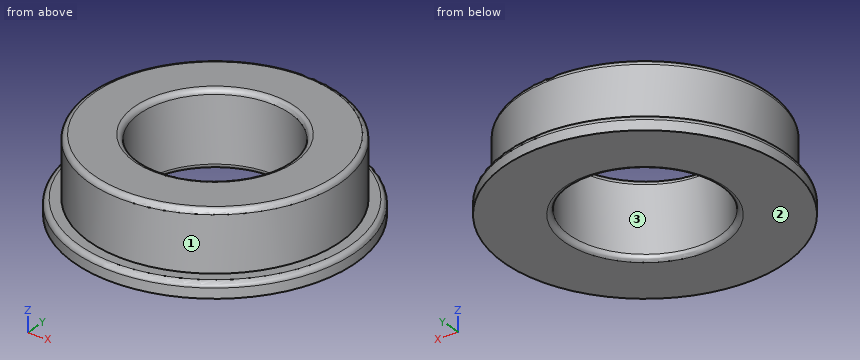
Autodesk Inventor part; units mm, degrees
ref_plane "YZ Plane" through (0, 0, 0) normal (1, 0, 0) x (0, 1, 0)
ref_plane "XZ Plane" through (0, 0, 0) normal (0, 1, 0) x (-1, 0, 0)
ref_plane "XY Plane" through (0, 0, 0) normal (0, 0, 1) x (1, 0, 0)
sketch "Sketch1" plane through (0, 0, 0) normal (0, 0, 1) x (1, 0, 0)
  circle A0 centre (0, 0) radius 3
  circle A1 centre (0, 0) radius 5
  circle A2 centre (0, 0) radius 5.6
  dimension "d0" = 6
  dimension "d1" = 10
  dimension "d2" = 11.2
extrude "Extrusion1" add sketch "Sketch1" along normal blind 3 contours A1
extrude "Extrusion2" add sketch "Sketch1" along normal blind 0.6 contours A2
fillet "Fillet1" radius 0.2 4 edges at (-5.6, 0, 0.6) (-5, 0, 3) (-3, 0, 3) (-3, 0, 0)
properties part number "flange_bearing"
Verification items for the finished model (mm, model axes). Face numbers are marked on the shaded views. Give positions to 0.01 mm unless a question says otherwise; leave off trailing zeros. Order: outer loops, then holes, each group sorted by start corner. A loop starts at its lowest first (then second) coordinate and runs counter-clockwise, first axis right, second up. Notation, with made-up numbers: (52, 39.5) -> (107, 39.5) arc R27 cw to (107, 59.5) -> close; hole circle Ø10 at (-6.5, -19). An arc over 180 degrees is marked (long way). Use a Markdown table: item, result.
1) Section check A-A, the plane x = 0. Record the boundary of the cut face in (y, z).
Results:
| item | result |
|---|---|
| outline | (-5.6, 0) -> (-3.2, 0) arc R0.2 ccw to (-3, 0.2) -> (-3, 2.8) arc R0.2 ccw to (-3.2, 3) -> (-4.8, 3) arc R0.2 ccw to (-5, 2.8) -> (-5, 0.6) -> (-5.4, 0.6) arc R0.2 ccw to (-5.6, 0.4) -> close; (3, 0.2) arc R0.2 ccw to (3.2, 0) -> (5.6, 0) -> (5.6, 0.4) arc R0.2 ccw to (5.4, 0.6) -> (5, 0.6) -> (5, 2.8) arc R0.2 ccw to (4.8, 3) -> (3.2, 3) arc R0.2 ccw to (3, 2.8) -> close |
2) Material ranges on probe 1 along Y at (x, z) = (0, 0.9); probe 2 along X at (y, z) = (1, 1.1); probe 3 along Z at (x, y) = (-1.25, -5), recorded low to high.
Results:
| item | result |
|---|---|
| probe 1 | -5 to -3, 3 to 5 |
| probe 2 | -4.9 to -2.83, 2.83 to 4.9 |
| probe 3 | 0 to 0.6 |
3) Mould release check, pull along X, two halves, no side actions. Record for the marked faces 1, 2 and 3: pulls with the +X half, pulls with the -X half, needs draft (parallel to the pull), parting line crosses it, or undercut.
Results:
| item | result |
|---|---|
| face 1 | parting line crosses it |
| face 2 | needs draft |
| face 3 | undercut |
4) Depth check by flat-ended pin: pin 1 Ø5.5 at (x, y) = (-2, 2) entering from +Z. Enter the tip coordinate at first touch or a pass-through.
Results:
| item | result |
|---|---|
| pin 1 | z = 3 |
5) Section check C-C, the plane z = 2.55. Record the boundary of the cut face in (x, y), then the cut area to 3 significant figures.
Results:
| item | result |
|---|---|
| outline | circle Ø10 at (0, 0); hole circle Ø6 at (0, 0) |
| area | 50.3 mm² |
